Input: part model. Units: mm. Frame: model coordinates. Round coordinates to 2 decimals unless told otherwise and drop trailing zeros. Loops run counter-clockwise (first coordinate to the right, second up) from the corner with the lowest first, then second, coordinate; pieces in that order, holes last. Notation, with made-up numbers: (65.25, 24) - (111.25, 24) arc R14 ccw to (111.25, 32) - close; hole circle Ø8 at (-21, 53). An arc over 180 degrees is marked (long way). Write each question's results on one line, items separated by ' | '.
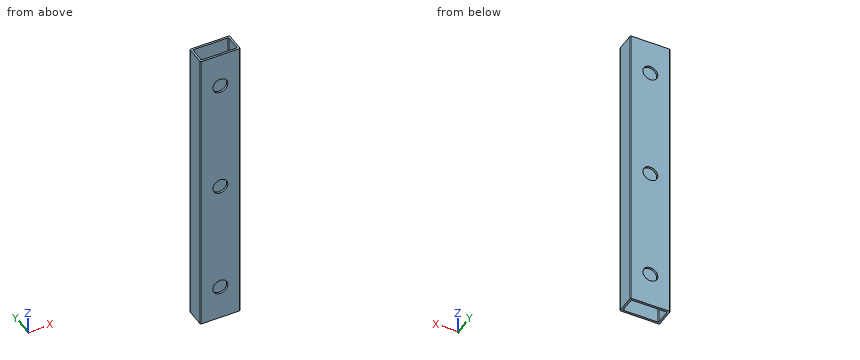
from build123d import *

# Parameters (mm, degrees)
BOSS_EXTRU_1_DEPTH      = 600
ESQUISSE2_R             = 15
ENL_V_MAT_EXTRU_1_DEPTH = 607.630035524


with BuildPart() as part:
    # Esquisse1 → Boss.-Extru.1 (new body)
    with BuildSketch(Plane.XY):
        with BuildLine():
            Line((2, -2), (78, -2))
            ThreePointArc((78, -2), (79.414213562, -1.414213562), (80, 0))
            Line((80, 0), (80, 36))
            ThreePointArc((80, 36), (79.414213562, 37.414213562), (78, 38))
            Line((78, 38), (2, 38))
            ThreePointArc((2, 38), (0.585786438, 37.414213562), (0, 36))
            Line((0, 36), (0, 0))
            ThreePointArc((0, 0), (0.585786438, -1.414213562), (2, -2))
        make_face()
        with BuildLine():
            Line((4, 4), (4, 32))
            ThreePointArc((4, 32), (4.585786438, 33.414213562), (6, 34))
            Line((6, 34), (74, 34))
            ThreePointArc((74, 34), (75.414213562, 33.414213562), (76, 32))
            Line((76, 32), (76, 4))
            ThreePointArc((76, 4), (75.414213562, 2.585786438), (74, 2))
            Line((74, 2), (6, 2))
            ThreePointArc((6, 2), (4.585786438, 2.585786438), (4, 4))
        make_face(mode=Mode.SUBTRACT)
    extrude(amount=BOSS_EXTRU_1_DEPTH)

    # Esquisse2 → Enlèv. mat.-Extru.1 (cut, through all)
    with BuildSketch(Plane(origin=(0, 38, 0), x_dir=(1, 0, 0), z_dir=(0, 1, 0))):
        with Locations(Location((40, -300, 0), (0, 0, 180))):
            Circle(ESQUISSE2_R)
        with Locations(Location((40, -70, 0), (0, 0, 180))):
            Circle(ESQUISSE2_R)
        with Locations(Location((40, -530, 0), (0, 0, 270))):
            Circle(ESQUISSE2_R)
    extrude(amount=-ENL_V_MAT_EXTRU_1_DEPTH, mode=Mode.SUBTRACT)


solid = part.part
1. Line query: line 1 (Y direction, x = 66.5, z = 329.5); line 2 (X direction, y = 36, z = 530); line 3 (X direction, y = 27.5, z = 409). Output: solid intervals per line, ascending. Write a range as [from, to].
Answer:
line 1: [-2, 2], [34, 38] | line 2: [0, 25], [55, 80] | line 3: [0, 4], [76, 80]
2. Section query D-D, the plane z = 229.5. Output: boundary loops of the cut face in (x, y), plus the area to 3 significant figures.
Answer:
outline: (0, 0) arc R2 ccw to (2, -2) - (78, -2) arc R2 ccw to (80, 0) - (80, 36) arc R2 ccw to (78, 38) - (2, 38) arc R2 ccw to (0, 36) - close; hole (4, 4) arc R2 ccw to (6, 2) - (74, 2) arc R2 ccw to (76, 4) - (76, 32) arc R2 ccw to (74, 34) - (6, 34) arc R2 ccw to (4, 32) - close | area: 896 mm^2
3. Section query A-A, the plane z = 70. Output: boundary loops of the cut face in (x, y), plus the area to 3 significant figures.
Answer:
outline: (0, 0) arc R2 ccw to (2, -2) - (25, -2) - (25, 2) - (6, 2) arc R2 cw to (4, 4) - (4, 32) arc R2 cw to (6, 34) - (25, 34) - (25, 38) - (2, 38) arc R2 ccw to (0, 36) - close; (55, -2) - (78, -2) arc R2 ccw to (80, 0) - (80, 36) arc R2 ccw to (78, 38) - (55, 38) - (55, 34) - (74, 34) arc R2 cw to (76, 32) - (76, 4) arc R2 cw to (74, 2) - (55, 2) - close | area: 656 mm^2
4. Section query B-B, the plane x = 40. Count the separate pieces of the cut face and the enclosed holes in it, plus the area to 3 significant figures.
Answer:
separate pieces: 8 | enclosed holes: 0 | area: 4,080 mm^2
5. Section query C-C, the plane y = 14. Output: boundary loops of the cut face in (x, z), plus the area to 3 significant figures.
Answer:
outline: (0, 0) - (4, 0) - (4, 600) - (0, 600) - close; (76, 0) - (80, 0) - (80, 600) - (76, 600) - close | area: 4,800 mm^2
